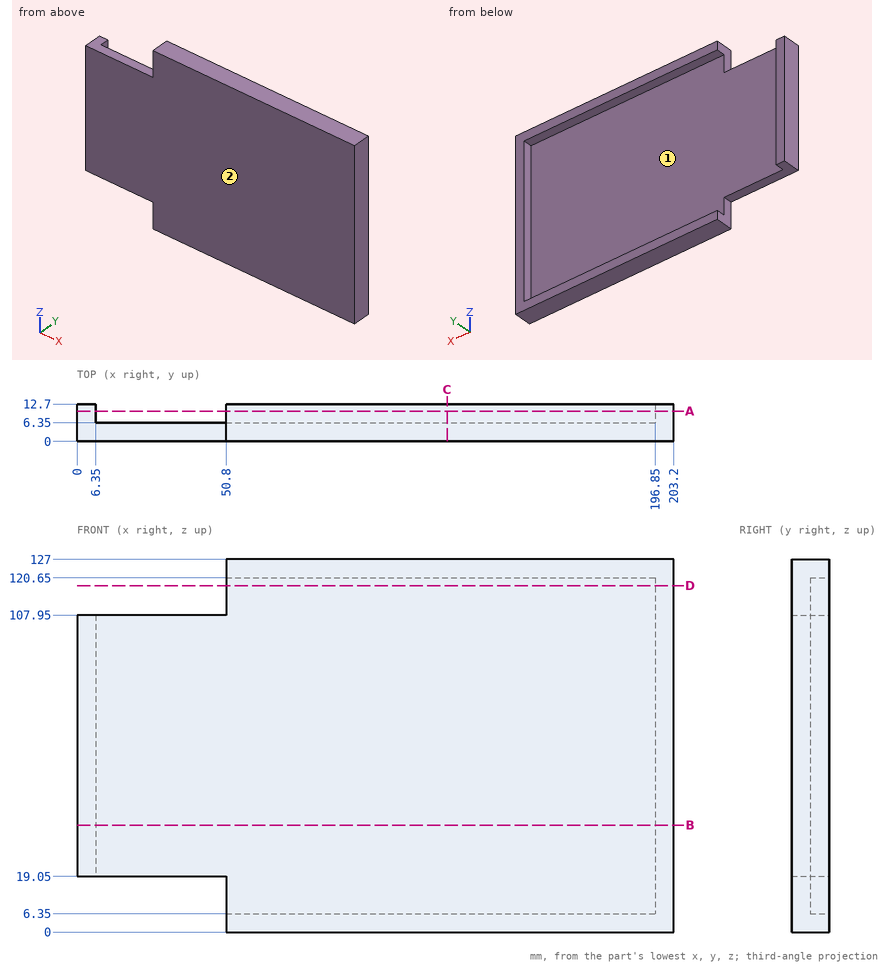
Geometry: see drawing. Coordinates: mm, zero at the bounding-box minimum. Coordinates: 2 decimals unless noted, no trailing zeros. Order: outer loops, then holes, each group sorted by start corner. A loop starts at its lowest first (then second) coordinate and runs counter-clockwise, first axis right, second up. Notation, with made-up numbers: M 82,74 L 92,74 A25 ccw 92,99 Z; hole C 53,78 d2. An arc over 180 degrees is marked long. Answer in a Markdown table with one row per item. Add a question column.
Q1. Section query B-B on z = 36.5. Return the cut outline in (x, y).
Q2. Mould query, pull axis X, two halves, no side actions, for the marked faces 1 and 2. Classes: released by +X, released by -X, zero draft, split by the parting line, or undercut.
Q3. Section query D-D on z = 118. Return the cut outline in (x, y).
Q4. Line query: L1, parallel to X at y = 10.5, z = 93; L2, parallel to Z at x = 175, y = 11; L3, parallel to Y at x = 181, z = 44. Output: solid intervals per line, ascending.
Q5. Section query C-C on x = 126. Return the cut outline in (y, z).
Q6. Contact query for a flat-ended pin moving along its axis: P1, Ø4, axis at x = 88.5, z = 109, coming from the +Y side. Output: stop coordinate, or through.
Q7. Section query A-A on y = 10.25. Return the cut outline in (x, z).
Completed:
| question | item | result |
|---|---|---|
| 1 | outline | M 0,0 L 203.2,0 L 203.2,12.7 L 196.85,12.7 L 196.85,6.35 L 6.35,6.35 L 6.35,12.7 L 0,12.7 Z |
| 2 | face 1 | undercut |
| 2 | face 2 | zero draft |
| 3 | outline | M 50.8,0 L 203.2,0 L 203.2,12.7 L 196.85,12.7 L 196.85,6.35 L 50.8,6.35 Z |
| 4 | L1 | x = 0 to 6.35, 196.85 to 203.2 |
| 4 | L2 | z = 0 to 6.35, 120.65 to 127 |
| 4 | L3 | y = 0 to 6.35 |
| 5 | outline | M 0,0 L 12.7,0 L 12.7,6.35 L 6.35,6.35 L 6.35,120.65 L 12.7,120.65 L 12.7,127 L 0,127 Z |
| 6 | P1 | stops at y = 6.35 |
| 7 | outline | M 0,19.05 L 6.35,19.05 L 6.35,107.95 L 0,107.95 Z; M 50.8,0 L 203.2,0 L 203.2,127 L 50.8,127 L 50.8,120.65 L 196.85,120.65 L 196.85,6.35 L 50.8,6.35 Z |
